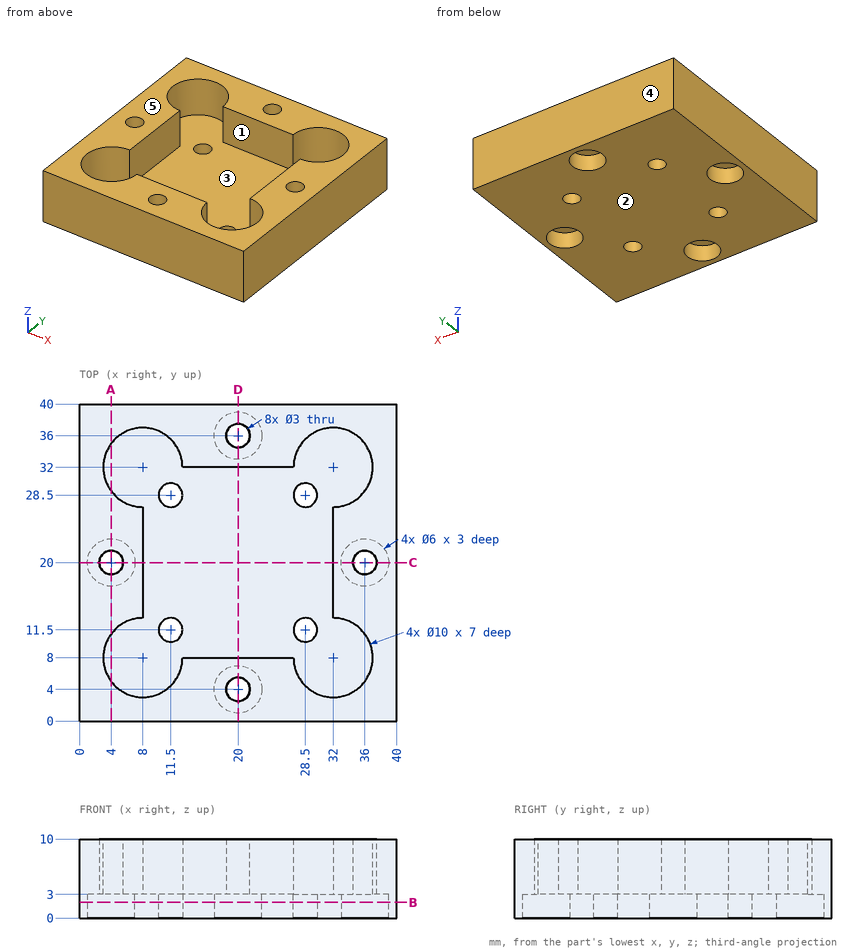
Verification items for this drawing (mm, ordinates from the low corner). A direction names the side the tool comes from. Coordinates: 2 decimals unless noted, no trailing zeros. Order: outer loops, then holes, each group sorted by start corner. A loop starts at its lowest first (then second) coordinate and runs counter-clockwise, first axis right, second up. Notation, with made-up numbers: (-28.5, -18) -> (3.5, -18) arc R31 ccw to (3.5, 14) -> close; hole circle Ø1 at (20.5, 84). An arc over 180 degrees is marked (long way). Answer as CSV lines item,"result". Start each with the question number.
1) Set-up check for the marked faces 1 and 2: record each of +Z, -Z, +X, -X, +Y, -Y from which the full face is reachable in a straight line by a thin tool's end or side.
2) Gauge pin test, flat ends, axial feed: pin 1 Ø5 at (x, y) = (21, 4) entering from -Z; pin 2 Ø10 at (x, y) = (18, 18.5) entering from +Z; pin 3 Ø5 at (x, y) = (4, 20) entering from -Z. Record the tip position at first contact, or that the pin passes through.
3) Cross-section at B-B, the plane z = 2. Give the number of separate pieces and of enclosed holes in the cut face, then the cut area to 3 significant figures.
4) Material ranges on L1, parallel to Y at x = 20, z = 1; L2, parallel to Y at x = 24, z = 8.75; L3, parallel to Y at x = 32.5, z = 6.5, recorded low to high. Write a range as [from, to].
5) Cross-section at C-C, the plane y = 20. Record the boundary of the cut face in (x, z).
6) Cross-section at A-A, the plane x = 4. Record the boundary of the cut face in (y, z).
7) Release check for a two-part mould opening along Y. For the marked faces 3, 4 and 5 record: released by +Y, released by -Y, zero draft, split by the parting line, or undercut.
Conclusion:
1,face 1,"+Z"
1,face 2,"-Z, +X, -X, +Y, -Y"
2,pin 1,"stops at z = 0"
2,pin 2,"stops at z = 3"
2,pin 3,"stops at z = 3"
3,separate pieces,"1"
3,enclosed holes,"8"
3,area,"1,460 mm²"
4,L1,"y = [0, 1], [7, 33], [39, 40]"
4,L2,"y = [0, 8], [32, 40]"
4,L3,"y = [0, 3.03], [12.97, 27.03], [36.97, 40]"
5,outline,"(0, 0) -> (1, 0) -> (1, 3) -> (2.5, 3) -> (2.5, 10) -> (0, 10) -> close; (5.5, 3) -> (7, 3) -> (7, 0) -> (33, 0) -> (33, 3) -> (34.5, 3) -> (34.5, 10) -> (32, 10) -> (32, 3) -> (8, 3) -> (8, 10) -> (5.5, 10) -> close; (37.5, 3) -> (39, 3) -> (39, 0) -> (40, 0) -> (40, 10) -> (37.5, 10) -> close"
6,outline,"(0, 0) -> (17, 0) -> (17, 3) -> (18.5, 3) -> (18.5, 10) -> (11, 10) -> (11, 3) -> (5, 3) -> (5, 10) -> (0, 10) -> close; (21.5, 3) -> (23, 3) -> (23, 0) -> (40, 0) -> (40, 10) -> (35, 10) -> (35, 3) -> (29, 3) -> (29, 10) -> (21.5, 10) -> close"
7,face 3,"undercut"
7,face 4,"released by +Y"
7,face 5,"zero draft"
